Here's the drawing with two shaded views (mm, measured from the low corner). I have some questions. A direction names the side the tool comes from. Coordinates: 2 decimals unless noted, no trailing zeros. Order: outer loops, then holes, each group sorted by start corner. A loop starts at its lowest first (then second) coordinate and runs counter-clockwise, first axis right, second up. Notation, with made-up numbers: (-27.5, 83.25) - (11.5, 83.25) arc R24 cw to (11.5, 99.25) - close; hole circle Ø3 at (4.25, 62.5). An arc over 180 degrees is marked (long way). Answer as CSV lines item,"result". Start each with the question number.
1. For pin 1 (12 mm diameter, centred on x = 41, z = 7.5, fed in from +Y); pin 2 (4 mm diameter, centred on x = 44.5, z = 5.5, fed in from -Y) (1 decimal); pin 3 (6 mm diameter, centred on y = 31.5, z = 17.5, fed in from -X), each with a flat end and sliding along its axis, tell me the tip position at first contact or that it passes through.
2. For the marked faces 1, 2 and 3, which set-ups out of +Z, -Z, +X, -X, +Y, -Y let a thin tool reach every point of the face, with its end or its side?
3. I want a section at B-B, the plane x = 39. List the corners of the cut face in (y, z) for me.
4. I need wall thicknesses on probe 1 along Y at (x, z) = (25.5, 24.75) (1 decimal); probe 2 along X at (y, z) = (22, 10.5) (1 decimal); probe 3 along X at (y, z) = (24, 9.75). Which ranges of each line are inside material? Lowest first, please.
5. I want a section at D-D, the plane x = 30. List the corners of the cut face in (y, z) for me, and give its area (3 significant figures).
6. Thinking about a two-plate mould opening in Y: for the marked faces 4, 5 and 6, which applies, released by +Y, released by -Y, zero draft, split by the parting line, or undercut?
7. I want a section at A-A, the plane y = 5.5. List the corners of the cut face in (x, z) for me (1 decimal).
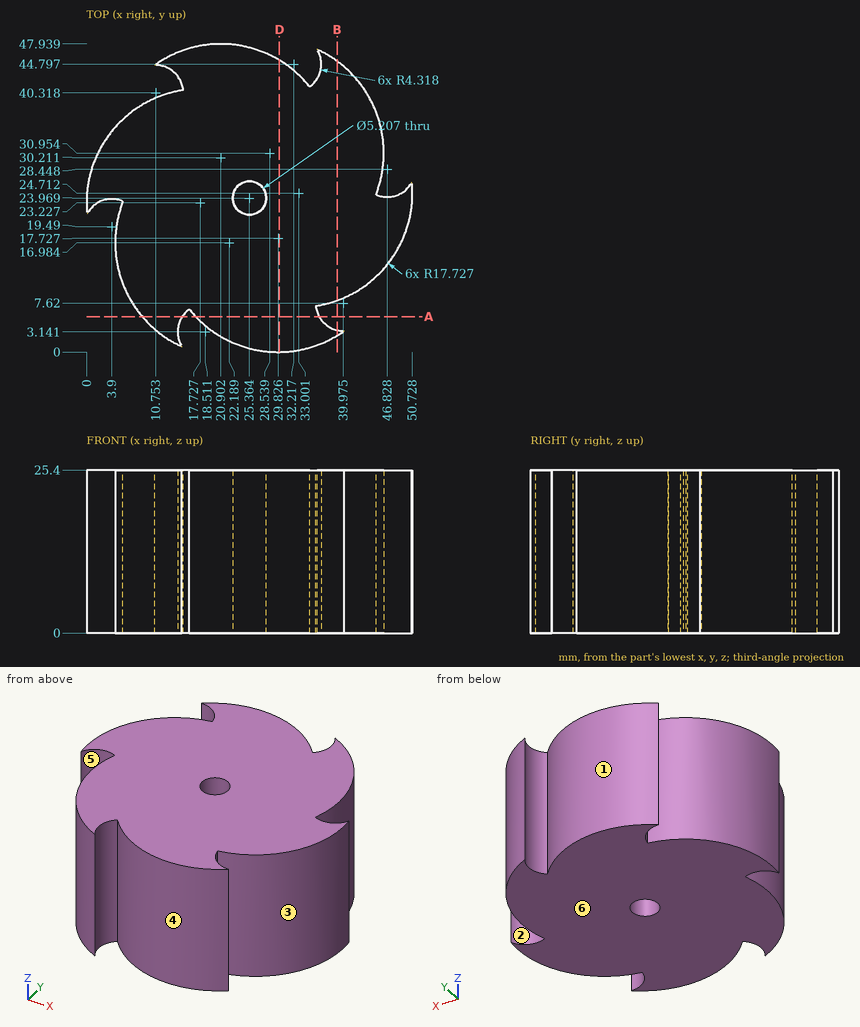
Solved:
1,pin 1,"stops at y = 47.09"
1,pin 2,"stops at y = 9.7"
1,pin 3,"stops at x = 0.8"
2,face 1,"+Z, -Z, +Y"
2,face 2,"+Z, -Z"
2,face 3,"+Z, -Z, +X"
3,outline,"(2.56, 0) - (3.41, 0) - (3.41, 25.4) - (2.56, 25.4) - close; (8.03, 0) - (45.27, 0) - (45.27, 25.4) - (8.03, 25.4) - close"
4,probe 1,"y = 0.5 to 21.4, 26.6 to 47.3"
4,probe 2,"x = 0 to 0.4, 5.2 to 23.7, 27.1 to 50.5"
4,probe 3,"x = 0.02 to 22.76, 27.97 to 50.71"
5,outline,"(0, 0) - (45.43, 0) - (45.43, 25.4) - (0, 25.4) - close"
5,area,"1,150 mm2"
6,face 4,"released by -Y"
6,face 5,"undercut"
6,face 6,"zero draft"
7,outline,"(8.7, 0) - (14.9, 0) - (14.9, 25.4) - (8.7, 25.4) - close; (17, 0) - (36.2, 0) - (36.2, 25.4) - (17, 25.4) - close"
